from build123d import *

# Parameters (mm, degrees)
SKETCH1_R           = 7.5
SKETCH1_R_2         = 5.15
BOSS_EXTRUDE1_DEPTH = 5
SKETCH1_3_R         = 5.15
BOSS_EXTRUDE2_DEPTH = 15.7
BOSS_EXTRUDE3_DEPTH = 4
SKETCH3_R           = 1.625
CUT_EXTRUDE1_DEPTH  = 37
SKETCH4_R           = 3.5
CUT_EXTRUDE2_DEPTH  = 10.7
BOSS_EXTRUDE4_START = 3.5
SKETCH5_R           = 7.5
SKETCH5_R_2         = 3.5
BOSS_EXTRUDE4_DEPTH = 3.5
BOSS_EXTRUDE5_START = 4
SKETCH6_R           = 15
SKETCH6_R_2         = 1.375
SKETCH6_R_3         = 3.5
BOSS_EXTRUDE5_DEPTH = 4
SKETCH7_R           = 3
CUT_EXTRUDE3_DEPTH  = 1
CUT_EXTRUDE4_START  = -12.5
SKETCH8_R           = 7.5
SKETCH8_R_2         = 7.45
CUT_EXTRUDE4_DEPTH  = 12.5
BOSS_EXTRUDE6_START = -8.5
SKETCH9_R           = 7.5
SKETCH9_R_2         = 7.45
BOSS_EXTRUDE6_DEPTH = 8.5
BOSS_EXTRUDE7_DEPTH = 4


with BuildPart() as part:
    # Sketch1 → Boss-Extrude1 (new body)
    # profile 1 of 2: a face of its own
    with BuildSketch(Plane(origin=(0, 0, 0), x_dir=(1, 0, 0), z_dir=(0, 1, 0))):
        with Locations(Location((0, 0, 0), (0, 0, 270))):
            Circle(SKETCH1_R)
        Circle(SKETCH1_R_2, mode=Mode.SUBTRACT)
    # profile 2 of 2: a face of its own
    with BuildSketch(Plane(origin=(0, 0, 0), x_dir=(1, 0, 0), z_dir=(0, 1, 0))):
        Circle(SKETCH1_R_2)
    extrude(amount=BOSS_EXTRUDE1_DEPTH)

    # Sketch1_3 → Boss-Extrude2 (add)
    with BuildSketch(Plane(origin=(0, 0, 0), x_dir=(1, 0, 0), z_dir=(0, 1, 0))):
        with Locations(Location((0, 0, 0), (0, 0, 270))):
            Circle(SKETCH1_3_R)
    extrude(amount=BOSS_EXTRUDE2_DEPTH)

    # Sketch2 → Boss-Extrude3 (add)
    with BuildSketch(Plane(origin=(0, 5, 0), x_dir=(1, 0, 0), z_dir=(0, 1, 0))):
        with BuildLine():
            ThreePointArc((7.5, 0), (5.303300859, 5.303300859), (0, 7.5))
            Line((0, 7.5), (0, 5.15))
            ThreePointArc((0, 5.15), (3.641599923, 3.641599923), (5.15, 0))
            ThreePointArc((5.15, 0), (3.641599923, -3.641599923), (0, -5.15))
            Line((0, -5.15), (0, -7.5))
            ThreePointArc((0, -7.5), (5.303300859, -5.303300859), (7.5, 0))
        make_face()
    extrude(amount=BOSS_EXTRUDE3_DEPTH)

    # Sketch3 → Cut-Extrude1 (cut)
    with BuildSketch(Plane.XZ):
        with Locations(Location((0, 0, 0), (0, 0, 270))):
            Circle(SKETCH3_R)
    extrude(amount=-CUT_EXTRUDE1_DEPTH, mode=Mode.SUBTRACT)

    # Sketch4 → Cut-Extrude2 (cut)
    with BuildSketch(Plane.XZ):
        with Locations(Location((0, 0, 0), (0, 0, 270))):
            Circle(SKETCH4_R)
    extrude(amount=-CUT_EXTRUDE2_DEPTH, mode=Mode.SUBTRACT)

    # Sketch5 → Boss-Extrude4 (add)
    with BuildSketch(Plane.XZ.offset(BOSS_EXTRUDE4_START)):
        with Locations(Location((0, 0, 0), (0, 0, 270))):
            Circle(SKETCH5_R)
        with Locations(Location((0, 0, 0), (0, 0, 270))):
            Circle(SKETCH5_R_2, mode=Mode.SUBTRACT)
    extrude(amount=-BOSS_EXTRUDE4_DEPTH)

    # Sketch6 → Boss-Extrude5 (add)
    with BuildSketch(Plane.XZ.offset(3.5).offset(BOSS_EXTRUDE5_START)):
        with Locations(Location((0, 0, 0), (0, 0, 270))):
            Circle(SKETCH6_R)
        with Locations(Location((11, 0, 0), (0, 0, 270))):
            Circle(SKETCH6_R_2, mode=Mode.SUBTRACT)
        with Locations(Location((7.778174593, -7.778174593, 0), (0, 0, 270))):
            Circle(SKETCH6_R_2, mode=Mode.SUBTRACT)
        with Locations(Location((0, -11, 0), (0, 0, 270))):
            Circle(SKETCH6_R_2, mode=Mode.SUBTRACT)
        with Locations(Location((-7.778174593, -7.778174593, 0), (0, 0, 270))):
            Circle(SKETCH6_R_2, mode=Mode.SUBTRACT)
        with Locations(Location((-11, 0, 0), (0, 0, 270))):
            Circle(SKETCH6_R_2, mode=Mode.SUBTRACT)
        with Locations(Location((-7.778174593, 7.778174593, 0), (0, 0, 270))):
            Circle(SKETCH6_R_2, mode=Mode.SUBTRACT)
        with Locations(Location((0, 11, 0), (0, 0, 270))):
            Circle(SKETCH6_R_2, mode=Mode.SUBTRACT)
        with Locations(Location((7.778174593, 7.778174593, 0), (0, 0, 270))):
            Circle(SKETCH6_R_2, mode=Mode.SUBTRACT)
        with Locations(Location((0, 0, 0), (0, 0, 270))):
            Circle(SKETCH6_R_3, mode=Mode.SUBTRACT)
    extrude(amount=-BOSS_EXTRUDE5_DEPTH)

    # Sketch7 → Cut-Extrude3 (cut)
    with BuildSketch(Plane(origin=(0, -3.5, 0), x_dir=(1, 0, 0), z_dir=(0, 1, 0))):
        with Locations(Location((-11, 0, 0), (0, 0, 270))):
            Circle(SKETCH7_R)
        with Locations(Location((-7.778174593, 7.778174593, 0), (0, 0, 270))):
            Circle(SKETCH7_R)
        with Locations(Location((0, 11, 0), (0, 0, 270))):
            Circle(SKETCH7_R)
        with Locations(Location((7.778174593, 7.778174593, 0), (0, 0, 270))):
            Circle(SKETCH7_R)
        with Locations(Location((11, 0, 0), (0, 0, 270))):
            Circle(SKETCH7_R)
        with Locations(Location((7.778174593, -7.778174593, 0), (0, 0, 270))):
            Circle(SKETCH7_R)
        with Locations(Location((0, -11, 0), (0, 0, 270))):
            Circle(SKETCH7_R)
        with Locations(Location((-7.778174593, -7.778174593, 0), (0, 0, 270))):
            Circle(SKETCH7_R)
    extrude(amount=-CUT_EXTRUDE3_DEPTH, mode=Mode.SUBTRACT)

    # Sketch8 → Cut-Extrude4 (cut)
    with BuildSketch(Plane(origin=(0, 9, 0), x_dir=(1, 0, 0), z_dir=(0, 1, 0)).offset(CUT_EXTRUDE4_START)):
        Circle(SKETCH8_R)
        with Locations(Location((0, 0, 0), (0, 0, 270))):
            Circle(SKETCH8_R_2, mode=Mode.SUBTRACT)
    extrude(amount=CUT_EXTRUDE4_DEPTH, mode=Mode.SUBTRACT)

    # Sketch9 → Boss-Extrude6 (add)
    with BuildSketch(Plane(origin=(0, 5, 0), x_dir=(1, 0, 0), z_dir=(0, 1, 0)).offset(BOSS_EXTRUDE6_START)):
        with Locations(Location((0, 0, 0), (0, 0, 270))):
            Circle(SKETCH9_R)
        Circle(SKETCH9_R_2, mode=Mode.SUBTRACT)
    extrude(amount=BOSS_EXTRUDE6_DEPTH)

    # Sketch10 → Boss-Extrude7 (add)
    with BuildSketch(Plane(origin=(0, 5, 0), x_dir=(1, 0, 0), z_dir=(0, 1, 0))):
        with BuildLine():
            ThreePointArc((7.5, 0), (5.303300859, 5.303300859), (0, 7.5))
            Line((0, 7.5), (0, 7.45))
            ThreePointArc((0, 7.45), (5.26794552, 5.26794552), (7.45, 0))
            ThreePointArc((7.45, 0), (5.26794552, -5.26794552), (0, -7.45))
            Line((0, -7.45), (0, -7.5))
            ThreePointArc((0, -7.5), (5.303300859, -5.303300859), (7.5, 0))
        make_face()
    extrude(amount=BOSS_EXTRUDE7_DEPTH)


solid = part.part
Here's how the part is built. I have some questions about the finished solid (model axes, mm). A direction names the side the tool comes from. Coordinates: 2 decimals unless noted, no trailing zeros. Order: outer loops, then holes, each group sorted by start corner. A loop starts at its lowest first (then second) coordinate and runs counter-clockwise, first axis right, second up.
Item 1: For faces 1 (the face through (0.1, -3.5, -7.7)), 2 (the face through (-3.417, 1.473, 0.759)), 3 (the face through (0, 7, -6)), which set-ups out of +Z, -Z, +X, -X, +Y, -Y let a thin tool reach every point of the face, with its end or its side?
Result sheet:
face 1: +Y
face 2: -Y
face 3: -Z, -X, +Y
Item 2: If we section it at B-B on z = 8.75: List the corners of the cut face in (x, y) for me.
Result sheet:
outline: (-12.18, -7.5) - (-8.75, -7.5) - (-8.75, -4.5) - (-10.62, -4.5) - (-10.62, -3.5) - (-12.18, -3.5) - close; (-6.81, -7.5) - (6.81, -7.5) - (6.81, -4.5) - (4.94, -4.5) - (4.94, -3.5) - (1.98, -3.5) - (1.98, -4.5) - (-1.98, -4.5) - (-1.98, -3.5) - (-4.94, -3.5) - (-4.94, -4.5) - (-6.81, -4.5) - close; (8.75, -7.5) - (12.18, -7.5) - (12.18, -3.5) - (10.62, -3.5) - (10.62, -4.5) - (8.75, -4.5) - close
Item 3: If we section it at D-D on x = 0.75: State how many separate pieces and enclosed holes the cut face has, plus the area to 3 significant figures.
Result sheet:
separate pieces: 4
enclosed holes: 0
area: 210 mm2
Item 4: For P1, Ø2, axis at y = 6.5, z = 4, coming from the +X side; P2, Ø4.5, axis at x = -7.78, z = -7.78, coming from the +Y side; P3, Ø2, axis at x = 3, y = -0.5, coming from the +Z side; P4, Ø3.5, axis at x = 0, z = 11, coming from the -Y side, each with a flat end and sliding along its axis, tell me the tip position at first contact or that it passes through.
Result sheet:
P1: stops at x = 6.87
P2: stops at y = -4.5
P3: stops at z = 7.23
P4: stops at y = -7.5
Item 5: I need wall thicknesses on line 1 (X direction, y = -5.1, z = 0) (3 decimals); line 2 (Y direction, x = -10.75, z = 9.75); line 3 (Y direction, x = -0.25, z = -2.5). Which ranges of each line are inside material? Lowest first, please.
Result sheet:
line 1: x = -15 to -12.375, -9.625 to -3.5, 3.5 to 9.625, 12.375 to 15
line 2: y = -7.5 to -3.5
line 3: y = 10.7 to 15.7
Item 6: If we mould it in two halves opening along Z, with no side actions, what happens to faces 4 (the face through (-10.1, -3.99, 2.86)), 5 (the face through (0, 7, 6)), 6 (the face through (-5.249, -3.993, -6.165))? For each: +Z half, -Z half, draft (parallel to the pull), parting line (faces both ways), or undercut.
Result sheet:
face 4: undercut
face 5: draft
face 6: undercut
Item 7: If we section it at A-A on x = 7: List the corners of the cut face in (y, z) for me, plus the area to 3 significant figures.
Result sheet:
outline: (-7.5, -13.27) - (-3.5, -13.27) - (-3.5, -10.68) - (-4.5, -10.68) - (-4.5, -8.91) - (-7.5, -8.91) - close; (-7.5, -6.64) - (-4.5, -6.64) - (-4.5, -4.88) - (-3.5, -4.88) - (-3.5, -2.69) - (9, -2.69) - (9, 2.69) - (-3.5, 2.69) - (-3.5, 4.88) - (-4.5, 4.88) - (-4.5, 6.64) - (-7.5, 6.64) - close; (-7.5, 8.91) - (-4.5, 8.91) - (-4.5, 10.68) - (-3.5, 10.68) - (-3.5, 13.27) - (-7.5, 13.27) - close
area: 148 mm2
Item 8: If we section it at C-C on z = 11.75: List the corners of the cut face in (x, y) for me, plus the area to 3 significant figures.
Result sheet:
outline: (-9.32, -7.5) - (-1.15, -7.5) - (-1.15, -4.5) - (-2.9, -4.5) - (-2.9, -3.5) - (-9.32, -3.5) - close; (1.15, -7.5) - (9.32, -7.5) - (9.32, -3.5) - (2.9, -3.5) - (2.9, -4.5) - (1.15, -4.5) - close
area: 61.9 mm2
